For this review, take the finished solid that the model builds, in its own axes (mm). A direction names the side the tool comes from. Coordinates: 2 decimals unless noted, no trailing zeros. Order: outer loops, then holes, each group sorted by start corner. A loop starts at its lowest first (then second) coordinate and runs counter-clockwise, first axis right, second up. Notation, with made-up numbers: (62, 78) -> (84, 78) arc R19 ccw to (84, 82) -> close; hole circle Ø6 at (5.25, -35.75). An arc over 180 degrees is marked (long way). Write item = value, one per line. Start each with the question number.
1) Consider section A-A on y = 0.5. Give the boundary of the cut face in (x, z), and give its area (3 significant figures).
2) Machinability: for faces 1 (the face through (3.045, -1.726, 2.958)), 2 (the face through (-3.955, -6.05, 1.944)), 3 (the face through (1.4, -7.2, 4)), which of the approach directions +Z, -Z, +X, -X, +Y, -Y give a long, thin tool a straight path to every point of the face, cutting with its end or side? Answer none if there is none.
3) Insertion check: pin 1 Ø4 at (x, y) = (0, 7.225) entering from -Z; pin 2 Ø3 at (x, y) = (0, -7.225) entering from +Z; pin 3 Ø2 at (y, z) = (2.5, 3) entering from -X; pin 4 Ø1 at (y, z) = (-2.5, 4) entering from -X. Each pin has a flat end and moves straight along its axis. Give the tip position at first contact, or say it passes through.
4) Wall thickness on probe 1 along Y at (x, z) = (0, 2.3) (3 decimals); probe 2 along Y at (x, z) = (0, -0.95) (3 decimals); probe 3 along Z at (x, y) = (-1, 8.75): over which ranges is each line inside the solid? List them lowest first. Write a range as [from, to].
5) Consider section C-C on z = 4.25. Give the boundary of the cut face in (x, y) (3 decimals), and give its area (3 significant figures).
6) Consider section D-D on y = 5.75. Give the boundary of the cut face in (x, z).
7) Draft analysis for pull direction Y (two halves, no side actions). For faces 4 (the face through (1.128, -10.425, 1.944)), 5 (the face through (-6.674, -0.037, 1.944)), 6 (the face through (1, 6, 4)), 7 (the face through (0, -3.5, 3)), state which applies: +Y half, -Y half, draft (parallel to the pull), parting line (faces both ways), or undercut.
8) Consider section B-B on x = -0.75. Give the boundary of the cut face in (y, z).
from build123d import *

# Parameters (mm, degrees)
F2_DEPTH      = 2
F7_DEPTH      = 6
F3_R          = 1.15
F8_DEPTH      = 2.001
F8_DEPTH_BACK = 6.001
F4_R          = 2.1
F9_DEPTH      = 2.001
F9_DEPTH_BACK = 4
F6_R          = 2.25
F10_DEPTH     = 2.001
F11_R         = 5
F12_R         = 2


with BuildPart() as f2:
    # F1 (on Top) → F2 (new body)
    with BuildSketch(Plane.XY):
        Polygon((1.2701705922, 10.7), (0, 10.7), (-1.2701705922, 10.7), (-7.4478184725, 0), (-1.2701705922, -10.7), (0, -10.7), (1.2701705922, -10.7), (7.4478184725, 0), align=None)
    extrude(amount=-F2_DEPTH)

    # F5 (on Top) → F7 (join)
    with BuildSketch(Plane.XY):
        Polygon((1.2701705922, -10.7), (7.4478184725, 0), (1.2701705922, 10.7), (0, 10.7), (-1.2701705922, 10.7), (-7.4478184725, 0), (-1.2701705922, -10.7), (0, -10.7), align=None)
        Polygon((2.0207259422, 3.5), (4.0414518843, 0), (2.0207259422, -3.5), (0, -3.5), (-2.0207259422, -3.5), (-4.0414518843, 0), (-2.0207259422, 3.5), (0, 3.5), align=None, mode=Mode.SUBTRACT)
    extrude(amount=F7_DEPTH)

    # F3 (on Top) → F8 (cut, two sides)
    with BuildSketch(Plane.XY) as f8_sk:
        with Locations((0, 7.225)):
            Circle(F3_R)
        with Locations((0, -7.225)):
            Circle(F3_R)
    extrude(amount=-F8_DEPTH, mode=Mode.SUBTRACT)
    extrude(f8_sk.sketch, amount=F8_DEPTH_BACK, mode=Mode.SUBTRACT)

    # F4 (on Top) → F9 (cut, two sides)
    with BuildSketch(Plane.XY) as f9_sk:
        with Locations((0, 7.225)):
            Circle(F4_R)
        with Locations((0, -7.225)):
            Circle(F4_R)
    extrude(amount=-F9_DEPTH, mode=Mode.SUBTRACT)
    extrude(f9_sk.sketch, amount=F9_DEPTH_BACK, mode=Mode.SUBTRACT)

    # F6 (on Top) → F10 (cut, through all)
    with BuildSketch(Plane.XY):
        Circle(F6_R)
    extrude(amount=-F10_DEPTH, mode=Mode.SUBTRACT)

    # F11
    f11_edges = [f2.edges().sort_by_distance(p)[0] for p in [
        (7.447818, 0, 2),
        (-7.447818, 0, 2),
    ]]
    fillet(f11_edges, radius=F11_R)

    # F12
    f12_edges = [f2.edges().sort_by_distance(p)[0] for p in [
        (1.270171, -10.7, 2),
        (-1.270171, -10.7, 2),
        (-1.270171, 10.7, 2),
        (1.270171, 10.7, 2),
    ]]
    fillet(f12_edges, radius=F12_R)


solid = f2.part
Answer sheet:
q1.outline = (-6.65, -2) -> (-2.19, -2) -> (-2.19, 0) -> (-3.75, 0) -> (-3.75, 6) -> (-6.65, 6) -> close; (2.19, -2) -> (6.65, -2) -> (6.65, 6) -> (3.75, 6) -> (3.75, 0) -> (2.19, 0) -> close
q1.area = 52.6 mm2
q2.face_1 = +Z
q2.face_2 = +Z, -Z, -X, -Y
q2.face_3 = -Z
q3.pin_1 = 4
q3.pin_2 = 6
q3.pin_3 = -6.44
q3.pin_4 = -6.26
q4.probe_1 = [-10.7, -9.325], [-5.125, -3.5], [3.5, 5.125], [9.325, 10.7]
q4.probe_2 = [-10.7, -9.325], [-5.125, -2.25], [2.25, 5.125], [9.325, 10.7]
q4.probe_3 = [4, 6]
q5.outline = (-6.004, -2.5) -> (-1.848, -9.7) arc R2 ccw to (-0.115, -10.7) -> (0.115, -10.7) arc R2 ccw to (1.848, -9.7) -> (6.004, -2.5) arc R5 ccw to (6.004, 2.5) -> (1.848, 9.7) arc R2 ccw to (0.115, 10.7) -> (-0.115, 10.7) arc R2 ccw to (-1.848, 9.7) -> (-6.004, 2.5) arc R5 ccw to start; hole (-4.041, 0) -> (-2.021, -3.5) -> (2.021, -3.5) -> (4.041, 0) -> (2.021, 3.5) -> (-2.021, 3.5) -> close; hole circle Ø2.3 at (0, -7.225); hole circle Ø2.3 at (0, 7.225)
q5.area = 132 mm2
q6.outline = (-4.13, -2) -> (-1.49, -2) -> (-1.49, 4) -> (1.49, 4) -> (1.49, -2) -> (4.13, -2) -> (4.13, 6) -> (-4.13, 6) -> close
q7.face_4 = -Y half
q7.face_5 = parting line
q7.face_6 = undercut
q7.face_7 = undercut
q8.outline = (-10.6, -2) -> (-9.19, -2) -> (-9.19, 4) -> (-8.1, 4) -> (-8.1, 6) -> (-10.6, 6) -> close; (-6.35, 4) -> (-5.26, 4) -> (-5.26, -2) -> (-2.12, -2) -> (-2.12, 0) -> (-3.5, 0) -> (-3.5, 6) -> (-6.35, 6) -> close; (2.12, -2) -> (5.26, -2) -> (5.26, 4) -> (6.35, 4) -> (6.35, 6) -> (3.5, 6) -> (3.5, 0) -> (2.12, 0) -> close; (8.1, 4) -> (9.19, 4) -> (9.19, -2) -> (10.6, -2) -> (10.6, 6) -> (8.1, 6) -> close
